```python
from build123d import *

# Parameters (mm, degrees)
SKETCH1_W           = 110
SKETCH1_H           = 140
SKETCH1_R           = 2
BOSS_EXTRUDE1_DEPTH = 5
SKETCH2_R           = 2
BOSS_EXTRUDE2_DEPTH = 5
SKETCH3_R           = 1.4732
SKETCH3_R_2         = 13
BOSS_EXTRUDE3_DEPTH = 5
BOSS_EXTRUDE4_DEPTH = 5


with BuildPart() as part:
    # Sketch1 → Boss-Extrude1 (new body)
    with BuildSketch(Plane.XY):
        Rectangle(SKETCH1_W, SKETCH1_H)
        with Locations((-47.5, 40)):
            Circle(SKETCH1_R, mode=Mode.SUBTRACT)
        with Locations((47.5, 40)):
            Circle(SKETCH1_R, mode=Mode.SUBTRACT)
        with Locations((-47.5, 60)):
            Circle(SKETCH1_R, mode=Mode.SUBTRACT)
        with Locations((47.5, 60)):
            Circle(SKETCH1_R, mode=Mode.SUBTRACT)
    extrude(amount=BOSS_EXTRUDE1_DEPTH)

    # Sketch2 → Boss-Extrude2 (add)
    with BuildSketch(Plane.XY):
        Polygon((-26.715730122, -70), (-55, -41.715730122), (-115, -101.715728753), (-115, -203), (-75, -203), (-75, -118.28427098), align=None)
        with Locations((-95, -185.5)):
            Circle(SKETCH2_R, mode=Mode.SUBTRACT)
        with Locations((-95, -150.5)):
            Circle(SKETCH2_R, mode=Mode.SUBTRACT)
    boss_extrude2 = extrude(amount=BOSS_EXTRUDE2_DEPTH)

    # Mirror1: Boss-Extrude2 across plane
    add(boss_extrude2.mirror(Plane(origin=(0, 0, 0), x_dir=(0, 0, 1), z_dir=(1, 0, 0))))

    # Sketch3 → Boss-Extrude3 (add)
    # profile 1 of 2: a face of its own
    with BuildSketch(Plane.XY.offset(5)):
        with BuildLine():
            ThreePointArc((-55, 49.531907673), (-151.188194001, 4.063503923), (-105.126050066, -91.841779044))
            Line((-105.126050066, -91.841779044), (-55, -41.715730122))
            Line((-55, -41.715730122), (-55, 49.531907673))
        make_face()
        with Locations((-143.929251903, 2.086359674)):
            Circle(SKETCH3_R, mode=Mode.SUBTRACT)
        with Locations((-92.221251993, 45.474523328)):
            Circle(SKETCH3_R, mode=Mode.SUBTRACT)
        with BuildLine():
            ThreePointArc((-65, -23), (-67, -21), (-65, -19))
            Line((-65, -19), (-61, -19))
            ThreePointArc((-61, -19), (-59, -21), (-61, -23))
            Line((-61, -23), (-65, -23))
        make_face(mode=Mode.SUBTRACT)
        with BuildLine():
            Line((-78.5, -40.5), (-82.5, -40.5))
            ThreePointArc((-82.5, -40.5), (-84.5, -38.5), (-82.5, -36.5))
            Line((-82.5, -36.5), (-78.5, -36.5))
            ThreePointArc((-78.5, -36.5), (-76.5, -38.5), (-78.5, -40.5))
        make_face(mode=Mode.SUBTRACT)
        with BuildLine():
            ThreePointArc((-96, -19), (-94, -21), (-96, -23))
            Line((-96, -23), (-100, -23))
            ThreePointArc((-100, -23), (-102, -21), (-100, -19))
            Line((-100, -19), (-96, -19))
        make_face(mode=Mode.SUBTRACT)
        with Locations((-80.5, -21)):
            Circle(SKETCH3_R_2, mode=Mode.SUBTRACT)
        with BuildLine():
            ThreePointArc((-82.5, -5.5), (-84.5, -3.5), (-82.5, -1.5))
            Line((-82.5, -1.5), (-78.5, -1.5))
            ThreePointArc((-78.5, -1.5), (-76.5, -3.5), (-78.5, -5.5))
            Line((-78.5, -5.5), (-82.5, -5.5))
        make_face(mode=Mode.SUBTRACT)
    # profile 2 of 2: a face of its own
    with BuildSketch(Plane.XY.offset(5)):
        with BuildLine():
            ThreePointArc((105.126050066, -91.841779044), (151.188194001, 4.063503923), (55, 49.531907673))
            Line((55, 49.531907673), (55, -41.715730122))
            Line((55, -41.715730122), (105.126050066, -91.841779044))
        make_face()
        with Locations((143.929251903, 2.086359674)):
            Circle(SKETCH3_R, mode=Mode.SUBTRACT)
        with Locations((92.221251993, 45.474523328)):
            Circle(SKETCH3_R, mode=Mode.SUBTRACT)
        with BuildLine():
            ThreePointArc((82.5, -1.5), (84.5, -3.5), (82.5, -5.5))
            Line((82.5, -5.5), (78.5, -5.5))
            ThreePointArc((78.5, -5.5), (76.5, -3.5), (78.5, -1.5))
            Line((78.5, -1.5), (82.5, -1.5))
        make_face(mode=Mode.SUBTRACT)
        with BuildLine():
            ThreePointArc((65, -19), (67, -21), (65, -23))
            Line((65, -23), (61, -23))
            ThreePointArc((61, -23), (59, -21), (61, -19))
            Line((61, -19), (65, -19))
        make_face(mode=Mode.SUBTRACT)
        with BuildLine():
            ThreePointArc((82.5, -36.5), (84.5, -38.5), (82.5, -40.5))
            Line((82.5, -40.5), (78.5, -40.5))
            ThreePointArc((78.5, -40.5), (76.5, -38.5), (78.5, -36.5))
            Line((78.5, -36.5), (82.5, -36.5))
        make_face(mode=Mode.SUBTRACT)
        with Locations((80.5, -21)):
            Circle(SKETCH3_R_2, mode=Mode.SUBTRACT)
        with BuildLine():
            Line((100, -23), (96, -23))
            ThreePointArc((96, -23), (94, -21), (96, -19))
            Line((96, -19), (100, -19))
            ThreePointArc((100, -19), (102, -21), (100, -23))
        make_face(mode=Mode.SUBTRACT)
    extrude(amount=-BOSS_EXTRUDE3_DEPTH)

    # Sketch4 → Boss-Extrude4 (add)
    with BuildSketch(Plane.XY.offset(5)):
        with BuildLine():
            Line((-170, -90), (-115, -203))
            Line((-115, -203), (-115, -157.300297485))
            Line((-115, -157.300297485), (-147.756781962, -90))
            Line((-147.756781962, -90), (-115, -90))
            Line((-115, -90), (-115, -101.715728753))
            Line((-115, -101.715728753), (-100, -101.715728753))
            Line((-100, -101.715728753), (-100, -90))
            Line((-100, -90), (-100, -40))
            Line((-100, -40), (-153.053428589, -40))
            ThreePointArc((-153.053428589, -40), (-155.304162069, -15.583604777), (-149.559478858, 8.253860938))
            Line((-149.559478858, 8.253860938), (-170, -40))
            Line((-170, -40), (-170, -90))
        make_face()
        with BuildLine():
            Line((-157.5, -54.55), (-162.5, -54.55))
            ThreePointArc((-162.5, -54.55), (-164.55, -52.5), (-162.5, -50.45))
            Line((-162.5, -50.45), (-157.5, -50.45))
            ThreePointArc((-157.5, -50.45), (-155.45, -52.5), (-157.5, -54.55))
        make_face(mode=Mode.SUBTRACT)
        with BuildLine():
            Line((-157.5, -75.45), (-162.5, -75.45))
            ThreePointArc((-162.5, -75.45), (-164.55, -77.5), (-162.5, -79.55))
            Line((-162.5, -79.55), (-157.5, -79.55))
            ThreePointArc((-157.5, -79.55), (-155.45, -77.5), (-157.5, -75.45))
        make_face(mode=Mode.SUBTRACT)
    boss_extrude4 = extrude(amount=-BOSS_EXTRUDE4_DEPTH)

    # Mirror2: Boss-Extrude4 across plane
    add(boss_extrude4.mirror(Plane(origin=(0, 0, 0), x_dir=(0, 0, 1), z_dir=(1, 0, 0))))


solid = part.part
```
Model file for the job. Use its own axes, mm. A direction names the side the tool comes from. Round coordinates to 2 decimals unless told otherwise and drop trailing zeros. Order: outer loops, then holes, each group sorted by start corner. A loop starts at its lowest first (then second) coordinate and runs counter-clockwise, first axis right, second up. Notation, with made-up numbers: M 7,-37.5 L 16,-37.5 A27 ccw 16,-5.5 Z; hole C -38.75,12 d7. An arc over 180 degrees is marked long. Use CSV: the item, a comma, the result in double quotes.
Item 1: Probe probe 1 along Y at (x, z) = (47.5, 3.3); probe 2 along X at (y, z) = (-108.5, 4.55); probe 3 along X at (y, z) = (-27, 1.1). List the from-to ranges inside material, lowest first.
Worked answers:
probe 1,"-90.78 to 38, 42 to 58, 62 to 70"
probe 2,"-161 to -138.75, -115 to -65.22, 65.22 to 115, 138.75 to 161"
probe 3,"-164.49 to -92.03, -68.97 to 68.97, 92.03 to 164.49"
Item 2: Saw through at C-C (x = 107). List the corners of the cut face in (y, z), plus the area to 3 significant figures.
Worked answers:
outline,"M -203,0 L 49.16,0 L 49.16,5 L -203,5 Z"
area,"1,260 mm²"
Item 3: Saw through at A-A (y = -12). List the corners of the cut face in (x, z).
Worked answers:
outline,"M -158.14,0 L -89.88,0 L -89.88,5 L -158.14,5 Z; M -71.12,0 L 71.12,0 L 71.12,5 L -71.12,5 Z; M 89.88,0 L 158.14,0 L 158.14,5 L 89.88,5 Z"
Item 4: Pin check, flat tips, straight feed: pin 1 (3 mm diameter, centred on x = 81.5, z = 2, fed in from +Y); pin 2 (1 mm diameter, centred on y = -150.5, z = 3.5, fed in from +X); pin 3 (1.8 mm diameter, centred on x = -92.22, y = 45.47, fed in from -Z); pin 4 (2.5 mm diameter, centred on y = 61, z = 3.5, fed in from +X). Stop position of each tip, or through.
Worked answers:
pin 1,"y = 54"
pin 2,"x = 140.8"
pin 3,"through"
pin 4,"x = 55"
Item 5: Which spindle directions (+Z, -Z, +X, -X, +Y, -Y) get a long thin tool onto all of the face, cutting with end or side? Do faces 5 (the face through (-51.196, -94.48, 2.465)), 6 (the face through (142.885, -145.709, 2.535)), 7 (the face through (-131.15, -124.12, 2.54)). Say none if no direction does.
Worked answers:
face 5,"+Z, -Z, -Y"
face 6,"+Z, -Z, +X, -Y"
face 7,"+Z, -Z"
Item 6: Pull direction X, two halves, no side cores. Call faces 1 (the face through (111.234, 47.414, 2.535)), 2 (the face through (159.64, -15.54, 2.54)), 3 (the face through (-142.885, -145.709, 2.535)), 4 (the face through (131.15, -124.12, 2.54)): released by +X, released by -X, zero draft, split by the parting line, or undercut.
Worked answers:
face 1,"undercut"
face 2,"released by +X"
face 3,"released by -X"
face 4,"undercut"
Item 7: Saw through at B-B (z = 1.85). State how many separate pieces and enclosed holes the cut face has, plus the area to 3 significant figures.
Worked answers:
separate pieces,"1"
enclosed holes,"28"
area,"56,900 mm²"
